Geometry: final body of the model. Coordinates: model frame, mm. Give positions to 0.01 mm unless a question says otherwise; leave off trailing zeros. Write each loop counter-clockwise with the first axis right and the second up, starting at its lowest first coordinate (ties: lowest second). Pieces come first, ordered by that corner, then holes. Notation, with made-up numbers: (3, 23) - (14, 23) arc R19 ccw to (14, 58) - close; hole circle Ø8 at (67, 78.5). An arc over 180 degrees is marked (long way). Use CSV: the item, a comma, the result in double quotes. Start each with the question number.
(1) Section B-B on y = -140. Output: boundary loops of the cut face in (x, z).
(2) Section C-C on z = 0.7. Count the separate pieces of the cut face and the enclosed holes in it, and give its area (3 significant figures).
(3) Section A-A on x = 60. Output: boundary loops of the cut face in (y, z), and give its area (3 significant figures).
(4) Line query: probe 1 along X at (y, z) = (-102, 1.1); probe 2 along X at (y, z) = (-140.5, 0.4); probe 3 along Y at (x, z) = (100, 0.6). Output: solid intervals per line, ascending. Write a range as [from, to].
(5) First-contact query: pin 1 Ø7 at (x, y) = (140, -20) entering from +Z; pin 2 Ø1 at (x, z) = (-71, 1.5) entering from -Y. Flat tips, straight axial feed; report the tip coordinate or a pass-through.
(6) Section D-D on x = -20. Output: boundary loops of the cut face in (y, z).
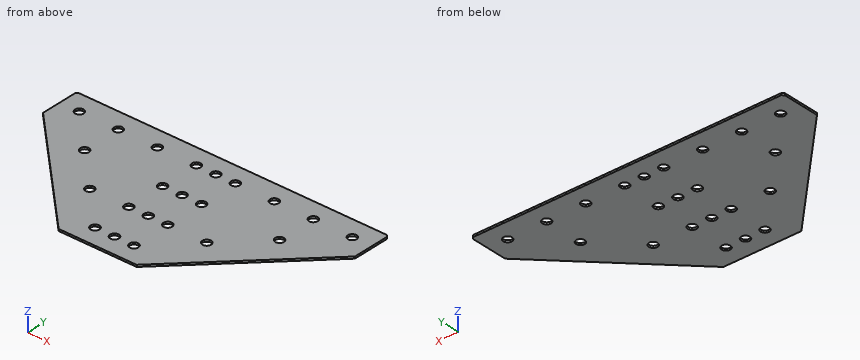
from build123d import *

# Parameters (mm, degrees)
EXTRUDE_1_DEPTH   = 2
CHAMFER_1_SIZE    = 2
HOLE_WIZARD_M81_D = 9


with BuildPart() as part:
    # Эскиз1 → Бобышка-Вытянуть1 (new body)
    with BuildSketch(Plane.XY):
        Polygon((160, -40), (40, -160), (-40, -160), (-160, -40), (-160, 0), (160, 0), align=None)
    extrude(amount=EXTRUDE_1_DEPTH)

    # Фаска1
    chamfer_1_edges = [part.edges().sort_by_distance(p)[0] for p in [
        (160, 0, 1),
        (-160, 0, 1),
    ]]
    chamfer(chamfer_1_edges, length=CHAMFER_1_SIZE)

    # Отверстие с зазором M81 (through all)
    with Locations(Plane.XY.offset(2)):
        with Locations((60, -100), (0, -20), (20, -20), (-20, -20), (-20, -60), (-20, -100), (-20, -140), (0, -60), (0, -100), (0, -140), (20, -60), (20, -100), (20, -140), (-60, -20), (-100, -20), (-140, -20), (60, -20), (100, -20), (140, -20), (-100, -60), (100, -60), (-60, -100)):
            Hole(HOLE_WIZARD_M81_D / 2)


solid = part.part
Check values:
1,outline,"(-60, 0) - (-24.5, 0) - (-24.5, 2) - (-60, 2) - close; (-15.5, 0) - (-4.5, 0) - (-4.5, 2) - (-15.5, 2) - close; (4.5, 0) - (15.5, 0) - (15.5, 2) - (4.5, 2) - close; (24.5, 0) - (60, 0) - (60, 2) - (24.5, 2) - close"
2,separate pieces,"1"
2,enclosed holes,"22"
2,area,"35,400 mm²"
3,outline,"(-140, 0) - (-104.5, 0) - (-104.5, 2) - (-140, 2) - close; (-95.5, 0) - (-24.5, 0) - (-24.5, 2) - (-95.5, 2) - close; (-15.5, 0) - (0, 0) - (0, 2) - (-15.5, 2) - close"
3,area,"244 mm²"
4,probe 1,"x = [-98, -64.03], [-55.97, -24.03], [-15.97, -4.03], [4.03, 15.97], [24.03, 55.97], [64.03, 98]"
4,probe 2,"x = [-59.5, -24.47], [-15.53, -4.47], [4.47, 15.53], [24.47, 59.5]"
4,probe 3,"y = [-100, -64.5], [-55.5, -24.5], [-15.5, 0]"
5,pin 1,"passes through"
5,pin 2,"stops at y = -129.5"
6,outline,"(-160, 0) - (-144.5, 0) - (-144.5, 2) - (-160, 2) - close; (-135.5, 0) - (-104.5, 0) - (-104.5, 2) - (-135.5, 2) - close; (-95.5, 0) - (-64.5, 0) - (-64.5, 2) - (-95.5, 2) - close; (-55.5, 0) - (-24.5, 0) - (-24.5, 2) - (-55.5, 2) - close; (-15.5, 0) - (0, 0) - (0, 2) - (-15.5, 2) - close"
